Answer from the drawing. Dimensions are ordinates in mm from the lowest x, y and z of the part. Coordinates: 2 decimals unless noted, no trailing zeros. Write each loop counter-clockwise with the first axis right and the second up, starting at its lowest first coordinate (ties: lowest second). Pieces come first, ordered by that corner, then holes.
(1) Given pin 1 (1.5 mm diameter, centred on y = 1.5, z = 1, fed in from +X); pin 2 (1.5 mm diameter, centred on x = 294, z = 1, fed in from +Y), each flat-ended and moving along its own axis, determine where each tip first touches the part or whether it passes through.
(2) The part is cut by section A-A, the plane z = 1.55. Determine the outline of the cut face in (x, y), and give its area (3 significant figures).
(3) A straight line is drawn through the part: line 1 along X through (y, z) = (10, 1.2). Find the intervals that lie inside material, in ascending order.
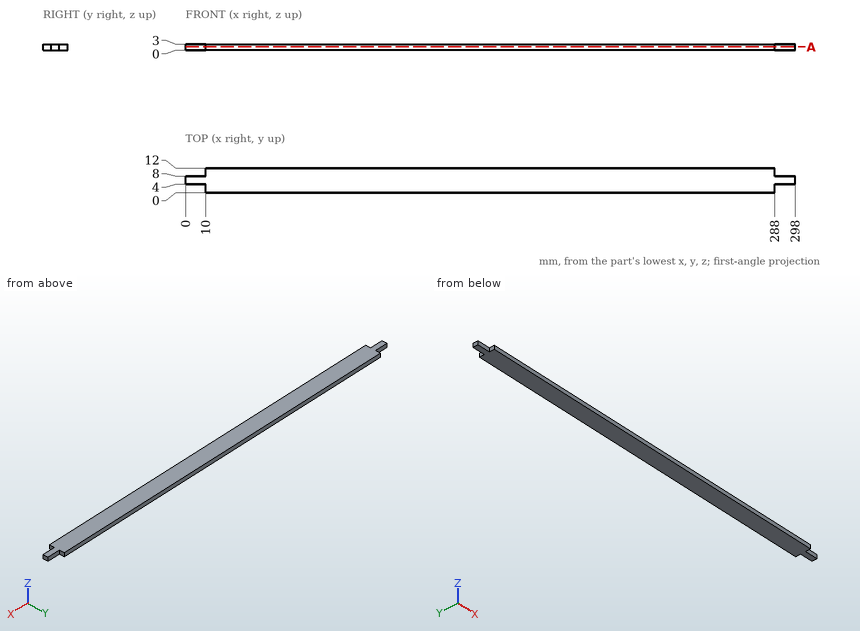
Computed:
1. pin 1: stops at x = 288
1. pin 2: stops at y = 8
2. outline: (0, 4) - (10, 4) - (10, 0) - (288, 0) - (288, 4) - (298, 4) - (298, 8) - (288, 8) - (288, 12) - (10, 12) - (10, 8) - (0, 8) - close
2. area: 3,420 mm2
3. line 1: x = 10 to 288
